```python
from build123d import *

# Parameters (mm, degrees)
F0_R     = 17.918738
F0_R_2   = 11.561225
F1_DEPTH = 25
F2_R     = 34.424869
F2_R_2   = 17.626187
F3_DEPTH = 61.5
F4_R     = 5
F5_SIZE  = 5
F6_SIZE  = 5
F7_R     = 5


with BuildPart() as f1:
    # F0 (on Front) → F1 (new body)
    with BuildSketch(Plane.XZ):
        with BuildLine():
            ThreePointArc((4.55913, -33.762444), (25.651635, -22.42057), (34.068876, 0))
            ThreePointArc((34.068876, 0), (25.85659, 22.183893), (5.178866, 33.672952))
            ThreePointArc((5.178866, 33.672952), (-34.067438, 0.313082), (4.55913, -33.762444))
        make_face()
        Circle(F0_R, mode=Mode.SUBTRACT)
        with BuildLine():
            ThreePointArc((5.178866, 33.672952), (25.85659, 22.183893), (34.068876, 0))
            ThreePointArc((34.068876, 0), (25.651635, -22.42057), (4.55913, -33.762444))
            Line((4.55913, -33.762444), (100.055945, -23.687435))
            ThreePointArc((100.055945, -23.687435), (73.738, -0.002993), (100.049991, 23.688063))
            Line((100.049991, 23.688063), (5.178866, 33.672952))
        make_face()
        with BuildLine():
            ThreePointArc((121.375793, 0), (115.25891, 15.936704), (100.049991, 23.688063))
            ThreePointArc((100.049991, 23.688063), (73.738, -0.002993), (100.055945, -23.687435))
            ThreePointArc((100.055945, -23.687435), (115.260913, -15.934479), (121.375793, 0))
        make_face()
        with Locations((97.556897, 0)):
            Circle(F0_R_2, mode=Mode.SUBTRACT)
    extrude(amount=F1_DEPTH)

    # F2 (on Front) → F3 (join)
    with BuildSketch(Plane.XZ):
        Circle(F2_R)
        Circle(F2_R_2, mode=Mode.SUBTRACT)
    extrude(amount=F3_DEPTH)

    # F4
    f4_edges = [f1.edges().sort_by_distance(p)[0] for p in [
        (-34.424869, -61.5, 0),
    ]]
    fillet(f4_edges, radius=F4_R)

    # F5
    f5_edges = [f1.edges().sort_by_distance(p)[0] for p in [
        (-17.626187, -61.5, 0),
    ]]
    chamfer(f5_edges, length=F5_SIZE)

    # F6
    f6_edges = [f1.edges().sort_by_distance(p)[0] for p in [
        (85.995671, -25, 0),
    ]]
    chamfer(f6_edges, length=F6_SIZE)

    # F7
    f7_edges = [f1.edges().sort_by_distance(p)[0] for p in [
        (54.318812, -25, -28.512748),
    ]]
    fillet(f7_edges, radius=F7_R)


solid = f1.part
```
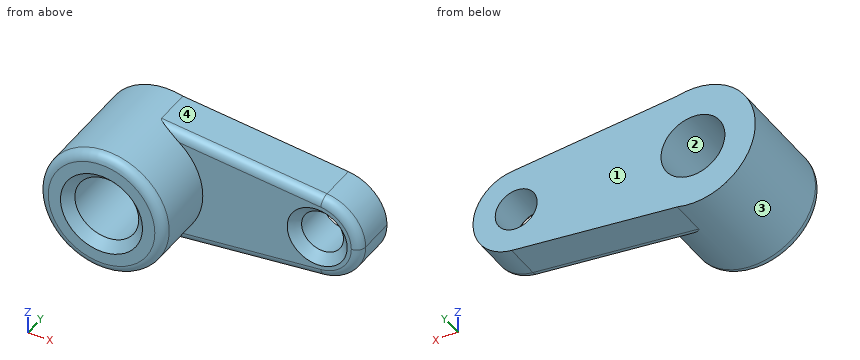
Source: CAD feature listing. Evaluate the final solid. Frame: model axes, mm. Face numbers are marked on the shaded views. Give positions to 0.01 mm unless a question says otherwise; leave off trailing zeros. Loops run counter-clockwise (first coordinate to the right, second up) from the corner with the lowest first, then second, coordinate; pieces in that order, holes last. Notation, with made-up numbers: (-23, 9) - (-1, 9) arc R24 cw to (-1, 47) - close; hole circle Ø3 at (-3, 81). An arc over 180 degrees is marked (long way). Use CSV: the item, a comma, the result in double quotes. Start each with the question number.
1. Section C-C (y = -29.5). Output: boundary loops of the cut face in (x, z).
2. Pin query (flat end, axial travel): pin 1 (5 mm diameter, centred on y = -31, z = -6.5, fed in from +X); pin 2 (8 mm diameter, centred on x = 83, z = 5, fed in from +Y); pin 3 (3 mm diameter, centred on x = 1, y = -8.5, fed in from -Z); pin 4 (6 mm diameter, centred on x = -14, y = -7.5, fed in from -Z). Return the tip coordinate at first contact, or that it passes through.
3. Section A-A (x = 0). Output: boundary loops of the cut face in (y, z), then the cut area to 3 significant figures.
4. Draft query along Z for the marked faces 1, 2, 3 and 4. Return one class per face: +Z half, -Z half, draft (parallel to the pull), parting line (faces both ways), or undercut.
5. Section B-B (y = -14.5). Output: boundary loops of the cut face in (x, z), then the cut area to 3 significant figures.
6. Ray query, L1, parallel to X at y = -11.5, z = 2; L2, parallel to Z at x = 0, y = -11.5; L3, parallel to Y at x = 45.5, z = -15.5. Return the intervals inside material, ascending.
Response:
1,outline,"circle Ø68.85 at (0, 0); hole circle Ø35.25 at (0, 0)"
2,pin 1,"x = 34.19"
2,pin 2,"y = 0"
2,pin 3,"z = -34.42"
2,pin 4,"z = -32.62"
3,outline,"(-61.5, -29.42) arc R5 ccw to (-56.5, -34.42) - (0, -34.42) - (0, -17.63) - (-56.5, -17.63) - (-61.5, -22.63) - close; (-61.5, 22.63) - (-56.5, 17.63) - (0, 17.63) - (0, 34.42) - (-56.5, 34.42) arc R5 ccw to (-61.5, 29.42) - close"
3,area,"2,030 mm²"
4,face 1,"draft"
4,face 2,"undercut"
4,face 3,"parting line"
4,face 4,"+Z half"
5,outline,"(8.58, -33.34) - (100.06, -23.69) arc R23.82 ccw to (121.38, 0) arc R23.82 ccw to (100.05, 23.69) - (8.73, 33.3) arc R34.42 ccw (long way) to start; hole circle Ø35.25 at (0, 0); hole circle Ø23.12 at (97.56, 0)"
5,area,"7,040 mm²"
6,L1,"-34.37 to -17.51, 17.51 to 86.17, 108.94 to 121.29"
6,L2,"-34.42 to -17.63, 17.63 to 34.42"
6,L3,"-25 to 0"
